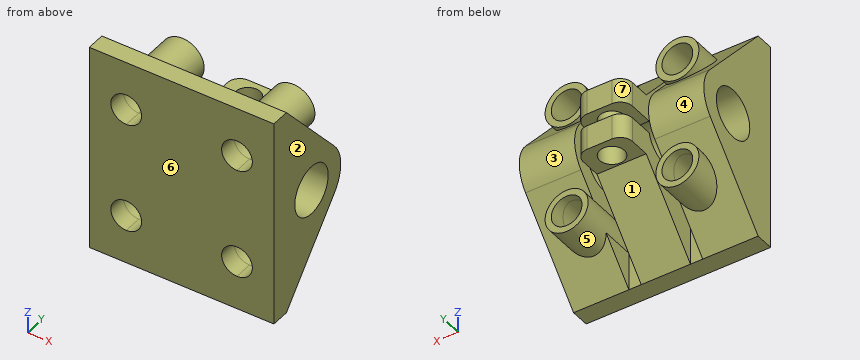
from build123d import *

# Parameters (mm, degrees)
SKETCH1_W           = 30
SKETCH1_H           = 34
SKETCH1_R           = 2.5
BOSS_EXTRUDE1_DEPTH = 3
SKETCH2_R           = 4
BOSS_EXTRUDE2_DEPTH = 30
SKETCH3_R           = 2.5
CUT_EXTRUDE1_DEPTH  = 49.082685508
SKETCH4_W           = 2
SKETCH4_H           = 13.407026696
CUT_EXTRUDE2_DEPTH  = 49.082685508
CUT_EXTRUDE3_REACH  = 44.106
SKETCH5_W           = 2
SKETCH5_H           = 4.553085987
SKETCH6_W           = 4
SKETCH6_H           = 6
SKETCH6_H_2         = 5.998001256
BOSS_EXTRUDE3_DEPTH = 8
SKETCH7_R           = 2
CUT_EXTRUDE4_DEPTH  = 42.715578629
FILLET1_R           = 2
SKETCH8_R           = 3.5
SKETCH8_R_2         = 2.5
BOSS_EXTRUDE4_DEPTH = 13.5


with BuildPart() as part:
    # Sketch1 → Boss-Extrude1 (new body)
    with BuildSketch(Plane(origin=(0, 0, 0), x_dir=(1, 0, 0), z_dir=(0, 1, 0))):
        with Locations((15, 17)):
            Rectangle(SKETCH1_W, SKETCH1_H)
        with Locations(Location((6, 26, 0), (0, 0, 270))):
            Circle(SKETCH1_R, mode=Mode.SUBTRACT)
        with Locations(Location((24, 26, 0), (0, 0, 270))):
            Circle(SKETCH1_R, mode=Mode.SUBTRACT)
        with Locations(Location((6, 8, 0), (0, 0, 270))):
            Circle(SKETCH1_R, mode=Mode.SUBTRACT)
        with Locations(Location((24, 8, 0), (0, 0, 270))):
            Circle(SKETCH1_R, mode=Mode.SUBTRACT)
    extrude(amount=BOSS_EXTRUDE1_DEPTH)

    # Sketch2 → Boss-Extrude2 (add, through all)
    with BuildSketch(Plane(origin=(30, 0, 0), x_dir=(0, 0, -1), z_dir=(1, 0, 0))):
        with BuildLine():
            Line((34, 3), (20.969729823, 14.497297215))
            ThreePointArc((20.969729823, 14.497297215), (17, 15.998270083), (13.030270177, 14.497297215))
            Line((13.030270177, 14.497297215), (0, 3))
            Line((0, 3), (34, 3))
        make_face()
        with Locations((17, 9)):
            Circle(SKETCH2_R, mode=Mode.SUBTRACT)
    extrude(amount=-BOSS_EXTRUDE2_DEPTH)

    # Sketch3 → Cut-Extrude1 (cut, through all)
    with BuildSketch(Plane.XZ):
        with Locations(Location((6, -8, 0), (0, 0, 90))):
            Circle(SKETCH3_R)
        with Locations(Location((24, -8, 0), (0, 0, 90))):
            Circle(SKETCH3_R)
        with Locations(Location((24, -26, 0), (0, 0, 270))):
            Circle(SKETCH3_R)
        with Locations(Location((6, -26, 0), (0, 0, 270))):
            Circle(SKETCH3_R)
    extrude(amount=-CUT_EXTRUDE1_DEPTH, mode=Mode.SUBTRACT)

    # Sketch4 → Cut-Extrude2 (cut, through all)
    with BuildSketch(Plane.XY):
        with Locations((10, 9.703513348)):
            Rectangle(SKETCH4_W, SKETCH4_H)
        with Locations((20, 9.703513348)):
            Rectangle(SKETCH4_W, SKETCH4_H)
    extrude(amount=-CUT_EXTRUDE2_DEPTH, mode=Mode.SUBTRACT)

    # Sketch5 → Cut-Extrude3 (cut, up to next)
    with BuildSketch(Plane.ZY.offset(-11), mode=Mode.PRIVATE) as cut_extrude3_sk1:
        with Locations((-17, 14.233519348)):
            Rectangle(SKETCH5_W, SKETCH5_H)
    cut_extrude3_tool1 = extrude(cut_extrude3_sk1.sketch, amount=-CUT_EXTRUDE3_REACH, mode=Mode.PRIVATE) & part.part
    add(cut_extrude3_tool1.solids().sort_by_distance((11, 14.233519, -17))[0], mode=Mode.SUBTRACT)

    # Sketch6 → Boss-Extrude3 (add)
    with BuildSketch(Plane.ZY.offset(-11)):
        with Locations((-14, 15.872983346)):
            Rectangle(SKETCH6_W, SKETCH6_H)
        with Locations((-20, 15.871983974)):
            Rectangle(SKETCH6_W, SKETCH6_H_2)
    extrude(amount=-BOSS_EXTRUDE3_DEPTH)

    # Sketch7 → Cut-Extrude4 (cut, through all)
    with BuildSketch(Plane.XY.offset(-12)):
        with Locations(Location((15, 15.872983346, 0), (0, 0, 90))):
            Circle(SKETCH7_R)
    extrude(amount=-CUT_EXTRUDE4_DEPTH, mode=Mode.SUBTRACT)

    # Fillet1
    fillet1_edges = [part.edges().sort_by_distance(p)[0] for p in [
        (19, 18.872983346, -14),
        (11, 18.872983346, -14),
        (19, 18.870984602, -20),
        (11, 18.870984602, -20),
    ]]
    fillet(fillet1_edges, radius=FILLET1_R)

    # Sketch8 → Boss-Extrude4 (add)
    # profile 1 of 4: a face of its own
    with BuildSketch(Plane(origin=(0, 0, 0), x_dir=(-1, 0, 0), z_dir=(0, -1, 0))):
        with Locations(Location((-6, 8, 0), (0, 0, 90))):
            Circle(SKETCH8_R)
        with Locations(Location((-6, 8, 0), (0, 0, 90))):
            Circle(SKETCH8_R_2, mode=Mode.SUBTRACT)
    # profile 2 of 4: a face of its own
    with BuildSketch(Plane(origin=(0, 0, 0), x_dir=(-1, 0, 0), z_dir=(0, -1, 0))):
        with Locations(Location((-24, 8, 0), (0, 0, 90))):
            Circle(SKETCH8_R)
        with Locations(Location((-24, 8, 0), (0, 0, 90))):
            Circle(SKETCH8_R_2, mode=Mode.SUBTRACT)
    # profile 3 of 4: a face of its own
    with BuildSketch(Plane(origin=(0, 0, 0), x_dir=(-1, 0, 0), z_dir=(0, -1, 0))):
        with Locations(Location((-6, 26, 0), (0, 0, 90))):
            Circle(SKETCH8_R)
        with Locations(Location((-6, 26, 0), (0, 0, 90))):
            Circle(SKETCH8_R_2, mode=Mode.SUBTRACT)
    # profile 4 of 4: a face of its own
    with BuildSketch(Plane(origin=(0, 0, 0), x_dir=(-1, 0, 0), z_dir=(0, -1, 0))):
        with Locations(Location((-24, 26, 0), (0, 0, 90))):
            Circle(SKETCH8_R)
        with Locations(Location((-24, 26, 0), (0, 0, 90))):
            Circle(SKETCH8_R_2, mode=Mode.SUBTRACT)
    extrude(amount=-BOSS_EXTRUDE4_DEPTH)


solid = part.part
Verification items for the finished model (mm, model axes). Face numbers are marked on the shaded views. A direction names the side the tool comes from. Coordinates: 2 decimals unless noted, no trailing zeros. Write each loop counter-clockwise with the first axis right and the second up, starting at its lowest first coordinate (ties: lowest second). Pieces come first, ordered by that corner, then holes. Notation, with made-up numbers: M 67.5,76 L 90.5,76 A24 ccw 90.5,100 Z; hole C 44.5,4 d1. An arc over 180 degrees is marked long. Use a Markdown table: item, result.
Q1. Sectioned sample at D-D, the plane x = 15. Record the boundary of the cut face in (y, z).
Reply:
| item | result |
|---|---|
| outline | M 0,-34 L 3,-34 L 13.59,-22 L 13.87,-22 L 13.87,-18 L 12.87,-18 A4 cw long 12.87,-16 L 13.87,-16 L 13.87,-12 L 13.59,-12 L 3,0 L 0,0 Z; M 17.87,-22 L 18.87,-22 L 18.87,-18 L 17.87,-18 Z; M 17.87,-16 L 18.87,-16 L 18.87,-12 L 17.87,-12 Z |
Q2. Go/stop test with flat-tipped pins: P1, Ø6, axis at x = 24, z = -8, coming from the +Y side; P2, Ø2, axis at x = 11, y = 13, coming from the +Z side; P3, Ø7.5, axis at x = 23, z = -8.5, coming from the +Y side; P4, Ø3.5, axis at x = 15, y = 15.87, coming from the -Z side. Record where each tip stops, or that it passes through.
Reply:
| item | result |
|---|---|
| P1 | stops at y = 13.5 |
| P2 | stops at z = -10.2 |
| P3 | stops at y = 13.81 |
| P4 | passes through |
Q3. Sectioned sample at C-C, the plane y = 9. Count the separate pieces of the cut face and the enclosed holes in it, plus the area to 3 significant figures.
Reply:
| item | result |
|---|---|
| separate pieces | 6 |
| enclosed holes | 4 |
| area | 292 mm² |
Q4. Sectioned sample at A-A, the plane z = -17. Record the boundary of the cut face in (x, y), plus the area to 3 significant figures.
Reply:
| item | result |
|---|---|
| outline | M 0,0 L 30,0 L 30,5 L 21,5 L 21,3 L 19,3 L 19,5 L 11,5 L 11,3 L 9,3 L 9,5 L 0,5 Z; M 0,13 L 9,13 L 9,16 L 0,16 Z; M 21,13 L 30,13 L 30,16 L 21,16 Z |
| area | 196 mm² |
Q5. Sectioned sample at B-B, the plane x = 24.75. Record the boundary of the cut face in (y, z), plus the area to 3 significant figures.
Reply:
| item | result |
|---|---|
| outline | M 0,-34 L 3,-34 L 7.04,-29.42 L 13.5,-29.42 L 13.5,-28.38 L 0,-28.38 Z; M 0,-23.62 L 13.5,-23.62 L 13.5,-22.58 L 13.08,-22.58 L 14.5,-20.97 A6 ccw 14.5,-13.03 L 13.08,-11.42 L 13.5,-11.42 L 13.5,-10.38 L 0,-10.38 Z; M 0,-5.62 L 13.5,-5.62 L 13.5,-4.58 L 7.04,-4.58 L 3,0 L 0,0 Z; hole C 9,-17 d8 |
| area | 219 mm² |
Q6. Set-up check for the marked faces 1, 2, 3 and 4: record each of +Z, -Z, +X, -X, +Y, -Y from which the full face is reachable in a straight line by a thin tool's end or side.
Reply:
| item | result |
|---|---|
| face 1 | -Z, +Y |
| face 2 | +Z, -Z, +X, +Y, -Y |
| face 3 | +X, +Y |
| face 4 | -X, +Y |
Q7. Thickness scan on line 1 (X direction, y = 5.25, z = -26); line 2 (X direction, y = 12.75, z = -26); line 3 (Z direction, x = 17.5, y = 15). Record the ranges inside material, lowest first.
Reply:
| item | result |
|---|---|
| line 1 | x = 0 to 3.5, 8.5 to 9.5, 11 to 19, 20.5 to 21.5, 26.5 to 30 |
| line 2 | x = 2.5 to 3.5, 8.5 to 9.5, 20.5 to 21.5, 26.5 to 27.5 |
| line 3 | z = -22 to -18, -16 to -12 |
Q8. Draft check along X on the marked faces 5, 6 and 7. Enter one of: +X half, -X half, draft (parallel to the pull), parting line (faces both ways), or undercut.
Reply:
| item | result |
|---|---|
| face 5 | undercut |
| face 6 | draft |
| face 7 | -X half |
